Model file for the job. Use its own axes, mm. Face numbers are marked on the shaded views. A direction names the side the tool comes from. Round coordinates to 2 decimals unless told otherwise and drop trailing zeros. Loops run counter-clockwise (first coordinate to the right, second up) from the corner with the lowest first, then second, coordinate; pieces in that order, holes last. Notation, with made-up numbers: (85.5, 39) -> (119.5, 39) arc R17 ccw to (119.5, 51) -> close; hole circle Ø2 at (73, 2.5). An arc over 180 degrees is marked (long way). Use a Markdown table: item, result.
from build123d import *

# Parameters (mm, degrees)
BOSS_EXTRUDE1_DEPTH = 50
FILLET1_R           = 2


with BuildPart() as part:
    # Sketch1 → Boss-Extrude1 (new body)
    with BuildSketch(Plane.XY):
        Polygon((-12.124355653, -7), (-3.464101615, 2), (0, 14), (3.464101615, 2), (12.124355653, -7), (0, -4), align=None)
    extrude(amount=BOSS_EXTRUDE1_DEPTH)

    # Fillet1
    fillet1_edges = [part.edges().sort_by_distance(p)[0] for p in [
        (-12.124355653, -7, 25),
        (0, 14, 25),
        (12.124355653, -7, 25),
    ]]
    fillet(fillet1_edges, radius=FILLET1_R)

    # Sketch2 → Cut-Revolve1 (revolve, cut)
    with BuildSketch(Plane(origin=(0, 0, 0), x_dir=(0, 0, -1), z_dir=(1, 0, 0))):
        Polygon((0, 8.788897449), (0, 3.788897449), (-14, 8.788897449), align=None)
    revolve(axis=Axis((0, 0, 0), (0, 0, -1)), mode=Mode.SUBTRACT)


solid = part.part
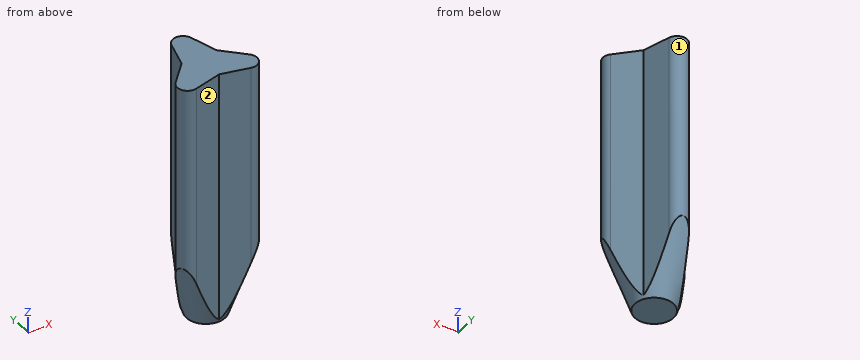
Q1. Tool access for the marked faces 1 and 2: list every direction of +Z, -Z, +X, -X, +Y, -Y with a clear straight run to the whole face (end or side of a thin tool).
Results list:
| item | result |
|---|---|
| face 1 | +Z, -Z, +Y |
| face 2 | +Z, -Z, -Y |
Q2. Flat gauge pins, fed straight in: pin 1 (1.5 mm diameter, centred on y = 5, z = 24, fed in from +X); pin 2 (1.5 mm diameter, centred on x = -4.5, y = 4, fed in from -Z). Where does each tip first touch, or does it go through?
Results list:
| item | result |
|---|---|
| pin 1 | stops at x = 2.81 |
| pin 2 | passes through |
Q3. Drill centre lines: L1, parallel to Y at x = 0, z = 24; L2, parallel to Y at x = 5, z = 35; L3, parallel to X at y = -0.5, z = 23.5. Where is each one in solid material? Low to high. Write a range as from..to.
Results list:
| item | result |
|---|---|
| L1 | y = -4..8.79 |
| L2 | y = -5.24..0.4 |
| L3 | x = -5.87..5.87 |
Q4. Band-saw the part on B-B, the plane y = 0. Give the cut face in (x, z), plus the area to 3 significant figures.
Results list:
| item | result |
|---|---|
| outline | (-5.39, 4.48) -> (-3.79, 0) -> (3.79, 0) -> (5.39, 4.48) -> (5.39, 50) -> (-5.39, 50) -> close |
| area | 532 mm² |
Q5. Band-saw the part on A-A, the plane z = 23. Give the cut face in (x, y).
Results list:
| item | result |
|---|---|
| outline | (-7.32, -2.01) arc R2 ccw to (-5.4, -5.34) -> (0, -4) -> (5.4, -5.34) arc R2 ccw to (7.32, -2.01) -> (3.46, 2) -> (1.92, 7.34) arc R2 ccw to (-1.92, 7.34) -> (-3.46, 2) -> close |
